Model file for the job. Use its own axes, mm. A direction names the side the tool comes from. Round coordinates to 2 decimals unless told otherwise and drop trailing zeros. Loops run counter-clockwise (first coordinate to the right, second up) from the corner with the lowest first, then second, coordinate; pieces in that order, holes last.
from build123d import *

# Parameters (mm, degrees)
SKETCH1_W           = 40
SKETCH1_H           = 20
SKETCH1_R           = 2.5
BOSS_EXTRUDE1_DEPTH = 20
SKETCH2_R           = 5
CUT_EXTRUDE1_DEPTH  = 18
SKETCH4_R           = 1.175
BOSS_EXTRUDE2_DEPTH = 6.4
FILLET1_R           = 0.5


with BuildPart() as part:
    # Sketch1 → Boss-Extrude1 (new body)
    with BuildSketch(Plane.XY):
        with Locations((5.224, 11.36)):
            Rectangle(SKETCH1_W, SKETCH1_H)
        with Locations((-4.776, 11.36)):
            Circle(SKETCH1_R, mode=Mode.SUBTRACT)
        with Locations((15.224, 11.36)):
            Circle(SKETCH1_R, mode=Mode.SUBTRACT)
    extrude(amount=BOSS_EXTRUDE1_DEPTH)

    # Sketch2 → Cut-Extrude1 (cut)
    with BuildSketch(Plane.XY.offset(20)):
        with Locations((-4.776, 11.36)):
            Circle(SKETCH2_R)
        with Locations((15.224, 11.36)):
            Circle(SKETCH2_R)
    extrude(amount=-CUT_EXTRUDE1_DEPTH, mode=Mode.SUBTRACT)

    # Sketch4 → Boss-Extrude2 (add)
    with BuildSketch(Plane(origin=(0, 21.36, 0), x_dir=(1, 0, 0), z_dir=(0, 1, 0))):
        with Locations(Location((9.974, -12.2, 0), (0, 0, 90))):
            Circle(SKETCH4_R)
        with Locations(Location((0.474, -12.2, 0), (0, 0, 90))):
            Circle(SKETCH4_R)
    extrude(amount=BOSS_EXTRUDE2_DEPTH)

    # Fillet1
    fillet1_edges = [part.edges().sort_by_distance(p)[0] for p in [
        (9.974, 27.76, 13.375),
        (0.474, 27.76, 13.375),
    ]]
    fillet(fillet1_edges, radius=FILLET1_R)


solid = part.part
Q1. Tool access for faces 5 (the face through (10.23, 11.58, 11.13)), 6 (the face through (0.422, 24.269, 13.374)), 7 (the face through (5, 12, 20)): list every direction of +Z, -Z, +X, -X, +Y, -Y with a clear straight run to the whole face (end or side of a thin tool).
Q2. Probe line 1 (X direction, y = 11.36, z = 1); line 2 (X direction, y = 12.25, z = 12); line 3 (Y direction, x = 6.5, z = 13.5). List the from-to ranges inside material, lowest first.
Q3. Slice it at D-D on x = 18.5. Give the cut face in (y, z).
Q4. Slice it at B-B on x = 14.5. Give the cut face in (y, z).
Q5. Flat gauge pins, fed straight in: P1, Ø5, axis at x = 16.5, y = 10, coming from the +Z side; P2, Ø4, axis at x = 6, z = 5, coming from the +Y side; P3, Ø3, axis at x = 15.224, y = 11.36, coming from the +Z side. Where does each tip first touch, or does it go through?
Q6. Slice it at A-A on z = 12.2. Give the cut face in (x, y).
Q7. Pull direction Y, two halves, no side cores. Call faces 1 (the face through (8.81, 24.27, 12.35)), 2 (the face through (12.726, 11.47, 0.986)), 3 (the face through (-5.32, 8.92, 0.99)), 4 (the face through (5, 1.36, 10)): pulls with the +Y half, pulls with the -Y half, needs draft (parallel to the pull), parting line crosses it, or undercut.
Q8. Slice it at C-C on y = 12. Give the cut face in (x, z).
Reply:
1. face 5: +Z
1. face 6: +Y
1. face 7: +Z, +X, -X, +Y, -Y
2. line 1: x = -14.78 to -7.28, -2.28 to 12.72, 17.72 to 25.22
2. line 2: x = -14.78 to -9.7, 0.14 to 10.3, 20.14 to 25.22
2. line 3: y = 1.36 to 21.36
3. outline: (1.36, 0) - (21.36, 0) - (21.36, 20) - (15.14, 20) - (15.14, 2) - (7.58, 2) - (7.58, 20) - (1.36, 20) - close
4. outline: (1.36, 0) - (8.97, 0) - (8.97, 2) - (6.41, 2) - (6.41, 20) - (1.36, 20) - close; (13.75, 0) - (21.36, 0) - (21.36, 20) - (16.31, 20) - (16.31, 2) - (13.75, 2) - close
5. P1: stops at z = 2
5. P2: stops at y = 21.36
5. P3: passes through
6. outline: (-14.78, 1.36) - (25.22, 1.36) - (25.22, 21.36) - (11.15, 21.36) - (11.15, 27.26) arc R0.5 ccw to (10.65, 27.76) - (9.3, 27.76) arc R0.5 ccw to (8.8, 27.26) - (8.8, 21.36) - (1.65, 21.36) - (1.65, 27.26) arc R0.5 ccw to (1.15, 27.76) - (-0.2, 27.76) arc R0.5 ccw to (-0.7, 27.26) - (-0.7, 21.36) - (-14.78, 21.36) - close; hole circle Ø10 at (-4.78, 11.36); hole circle Ø10 at (15.22, 11.36)
7. face 1: needs draft
7. face 2: undercut
7. face 3: undercut
7. face 4: pulls with the -Y half
8. outline: (-14.78, 0) - (-7.19, 0) - (-7.19, 2) - (-9.73, 2) - (-9.73, 20) - (-14.78, 20) - close; (-2.36, 0) - (12.81, 0) - (12.81, 2) - (10.27, 2) - (10.27, 20) - (0.18, 20) - (0.18, 2) - (-2.36, 2) - close; (17.64, 0) - (25.22, 0) - (25.22, 20) - (20.18, 20) - (20.18, 2) - (17.64, 2) - close
